Answer from the drawing. Dimensions are ordinates in mm from the lowest x, y and z of the part. A direction names the side the tool comes from. Coordinates: 2 decimals unless noted, no trailing zeros. Order: outer loops, then holes, each group sorted by start corner. A loop starts at its lowest first (then second) coordinate and runs counter-clockwise, first axis right, second up. Notation, with made-up numbers: (60, 35.5) - (92, 35.5) arc R26 ccw to (92, 66.5) - close; hole circle Ø2 at (8.25, 58). An arc over 180 degrees is marked (long way). Answer as a JSON object with one key per item and string values. Group by question number.
1) Section B-B (x = 178) is taken. Give the vertices of the cut face in (y, z), plus the area to 3 significant figures.
2) Section D-D (x = 110) is taken. Give the vertices of the cut face in (y, z).
3) Each of these flat-tipped pins is pushed along its axis until it touches: P1, Ø5, axis at x = 80, y = 16.5, coming from the -Z side; P2, Ø1.5, axis at x = 139, y = 70, coming from the +Z side; P3, Ø12, axis at y = 26.5, z = 10.5, coming from the +X side. Where does it stop, or does it pass through?
4) Find the intervals of material crossed by line 1 along X through (y, z) = (29, 13); line 2 along Y through (x, z) = (30, 31.5); line 3 along Z through (x, y) = (40, 58), in increasing order.
5) A tool of negligible diameter and unlimited length cuts with its end or side. For the marked faces 4, 5, 6, 7 and 8, from which of +Z, -Z, +X, -X, +Y, -Y can it reach the whole face along a straight path? Write none if from no direction.
6) The mould has two halves that part along Z. Classify the marked faces 1, 2 and 3: released by +Z, released by -Z, zero draft, split by the parting line, or undercut.
7) Section C-C (y = 41) is taken. Give the vertices of the cut face in (x, z), plus the area to 3 significant figures.
8) Section A-A (y = 64) is taken. Give the vertices of the cut face in (x, z), plus the area to 3 significant figures.
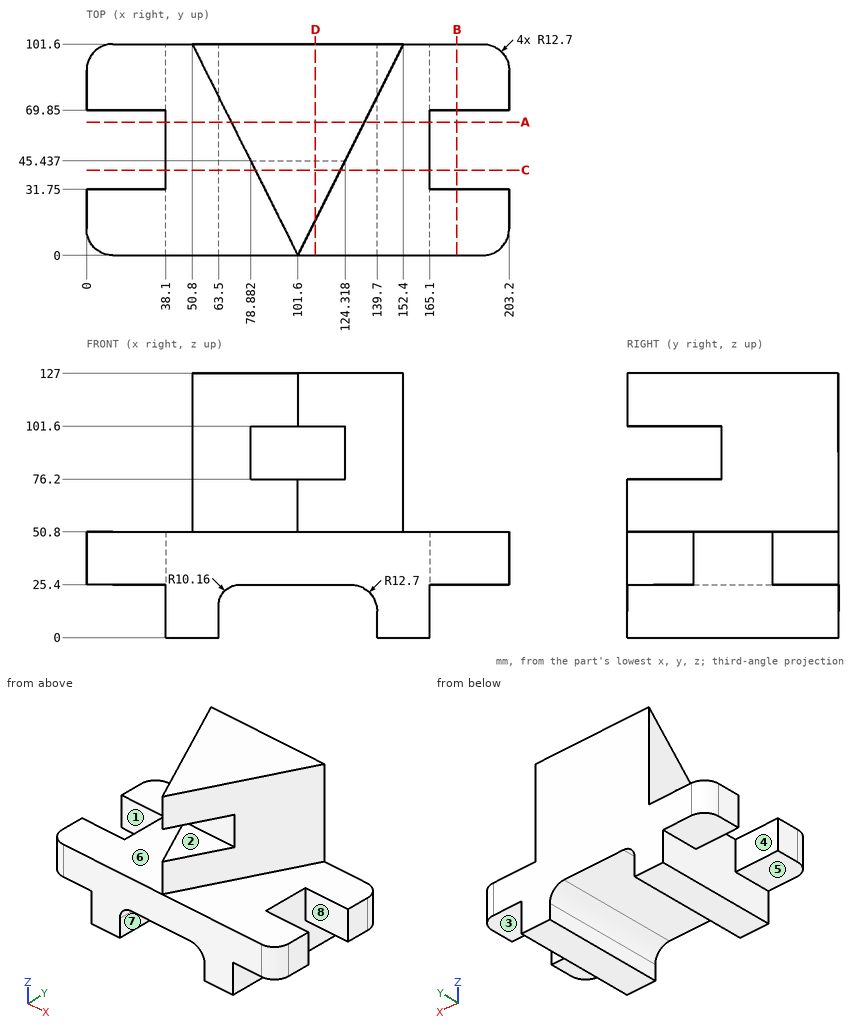
Report:
{
 "1": {"outline": "(0, 25.4) - (31.75, 25.4) - (31.75, 50.8) - (0, 50.8) - close; (69.85, 25.4) - (101.6, 25.4) - (101.6, 50.8) - (69.85, 50.8) - close", "area": "1,610 mm²"},
 "2": {"outline": "(0, 25.4) - (101.6, 25.4) - (101.6, 127) - (16.8, 127) - (16.8, 101.6) - (45.44, 101.6) - (45.44, 76.2) - (16.8, 76.2) - (16.8, 50.8) - (0, 50.8) - close"},
 "3": {"P1": "stops at z = 25.4", "P2": "stops at z = 50.8", "P3": "stops at x = 165.1"},
 "4": {"line 1": "x = 38.1 to 63.5, 139.7 to 165.1", "line 2": "y = 0 to 31.75, 69.85 to 101.6", "line 3": "z = 0 to 50.8"},
 "5": {"face 4": "+Z, -Z, -X", "face 5": "-Z, -X, +Y, -Y", "face 6": "+Z, -X, -Y", "face 7": "-Z, +Y, -Y", "face 8": "+Z, -Z, +X"},
 "6": {"face 1": "zero draft", "face 2": "undercut", "face 3": "released by -Z"},
 "7": {"outline": "(38.1, 0) - (63.5, 0) - (63.5, 15.24) arc R10.16 cw to (73.66, 25.4) - (127, 25.4) arc R12.7 cw to (139.7, 12.7) - (139.7, 0) - (165.1, 0) - (165.1, 50.8) - (122.1, 50.8) - (122.1, 76.2) - (81.1, 76.2) - (81.1, 50.8) - (38.1, 50.8) - close; (81.1, 101.6) - (122.1, 101.6) - (122.1, 127) - (81.1, 127) - close", "area": "6,660 mm²"},
 "8": {"outline": "(38.1, 0) - (63.5, 0) - (63.5, 15.24) arc R10.16 cw to (73.66, 25.4) - (127, 25.4) arc R12.7 cw to (139.7, 12.7) - (139.7, 0) - (165.1, 0) - (165.1, 50.8) - (133.6, 50.8) - (133.6, 127) - (69.6, 127) - (69.6, 50.8) - (38.1, 50.8) - close", "area": "9,450 mm²"}
}
